Can you work these out from the model? Positions are in its coordinate system, mm. Round coordinates to 2 decimals unless told otherwise and drop trailing zeros. Loops run counter-clockwise (first coordinate to the right, second up) from the corner with the lowest first, then second, coordinate; pieces in that order, holes last. Notation, with made-up numbers: M 24,22.5 L 40,22.5 A36 cw 40,56.5 Z; hole C 19,9 d8. An arc over 180 degrees is marked long. Return JSON: item names as keys, results as strings.
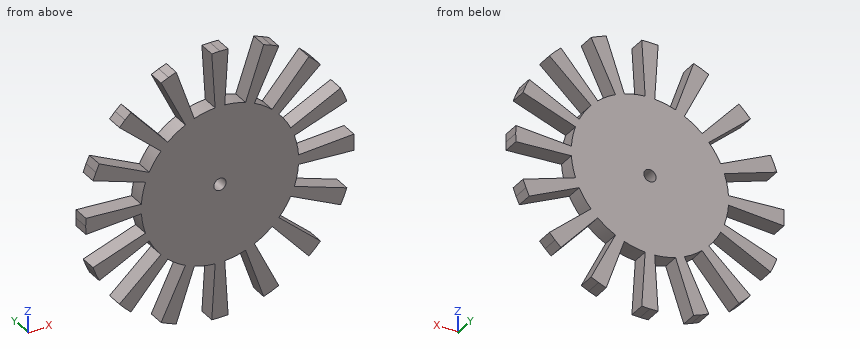
```python
from build123d import *

# Parameters (mm, degrees)
SKETCH2_R           = 1.89865
BOSS_EXTRUDE1_DEPTH = 5.1308


with BuildPart() as part:
    # Sketch2 → Boss-Extrude1 (new body)
    with BuildSketch(Plane(origin=(0, 0, 0), x_dir=(1, 0, 0), z_dir=(0, 1, 0))):
        with BuildLine():
            Line((-15.989661855, 38.602458507), (-13.614547531, 39.502698446))
            Line((-13.614547531, 39.502698446), (-7.982511303, 23.161308603))
            ThreePointArc((-7.982511303, 23.161308603), (-4.779381236, 24.027572035), (-1.488570263, 24.453033788))
            Line((-1.488570263, 24.453033788), (-2.538826421, 41.705796353))
            Line((-2.538826421, 41.705796353), (0, 41.783))
            Line((0, 41.783), (2.538826421, 41.705796353))
            Line((2.538826421, 41.705796353), (1.488570263, 24.453033788))
            ThreePointArc((1.488570263, 24.453033788), (4.779381236, 24.027572035), (7.982511303, 23.161308603))
            Line((7.982511303, 23.161308603), (13.614547531, 39.502698446))
            Line((13.614547531, 39.502698446), (15.989661855, 38.602458507))
            Line((15.989661855, 38.602458507), (18.305687065, 37.559564828))
            Line((18.305687065, 37.559564828), (10.733030501, 22.022006247))
            ThreePointArc((10.733030501, 22.022006247), (13.61052624, 20.369592003), (16.238327885, 18.34348414))
            Line((16.238327885, 18.34348414), (27.695230037, 31.285672794))
            Line((27.695230037, 31.285672794), (29.545042638, 29.545042638))
            Line((29.545042638, 29.545042638), (31.285672794, 27.695230037))
            Line((31.285672794, 27.695230037), (18.34348414, 16.238327885))
            ThreePointArc((18.34348414, 16.238327885), (20.369592003, 13.61052624), (22.022006247, 10.733030501))
            Line((22.022006247, 10.733030501), (37.559564828, 18.305687065))
            Line((37.559564828, 18.305687065), (38.602458507, 15.989661855))
            Line((38.602458507, 15.989661855), (39.502698446, 13.614547531))
            Line((39.502698446, 13.614547531), (23.161308603, 7.982511303))
            ThreePointArc((23.161308603, 7.982511303), (24.027572035, 4.779381236), (24.453033788, 1.488570263))
            Line((24.453033788, 1.488570263), (41.705796353, 2.538826421))
            Line((41.705796353, 2.538826421), (41.783, 0))
            Line((41.783, 0), (41.705796353, -2.538826421))
            Line((41.705796353, -2.538826421), (24.453033788, -1.488570263))
            ThreePointArc((24.453033788, -1.488570263), (24.027572035, -4.779381236), (23.161308603, -7.982511303))
            Line((23.161308603, -7.982511303), (39.502698446, -13.614547531))
            Line((39.502698446, -13.614547531), (38.602458507, -15.989661855))
            Line((38.602458507, -15.989661855), (37.559564828, -18.305687065))
            Line((37.559564828, -18.305687065), (22.022006247, -10.733030501))
            ThreePointArc((22.022006247, -10.733030501), (20.369592003, -13.61052624), (18.34348414, -16.238327885))
            Line((18.34348414, -16.238327885), (31.285672794, -27.695230037))
            Line((31.285672794, -27.695230037), (29.545042638, -29.545042638))
            Line((29.545042638, -29.545042638), (27.695230037, -31.285672794))
            Line((27.695230037, -31.285672794), (16.238327885, -18.34348414))
            ThreePointArc((16.238327885, -18.34348414), (13.61052624, -20.369592003), (10.733030501, -22.022006247))
            Line((10.733030501, -22.022006247), (18.305687065, -37.559564828))
            Line((18.305687065, -37.559564828), (15.989661855, -38.602458507))
            Line((15.989661855, -38.602458507), (13.614547531, -39.502698446))
            Line((13.614547531, -39.502698446), (7.982511303, -23.161308603))
            ThreePointArc((7.982511303, -23.161308603), (4.779381236, -24.027572035), (1.488570263, -24.453033788))
            Line((1.488570263, -24.453033788), (2.538826421, -41.705796353))
            Line((2.538826421, -41.705796353), (0, -41.783))
            Line((0, -41.783), (-2.538826421, -41.705796353))
            Line((-2.538826421, -41.705796353), (-1.488570263, -24.453033788))
            ThreePointArc((-1.488570263, -24.453033788), (-4.779381236, -24.027572035), (-7.982511303, -23.161308603))
            Line((-7.982511303, -23.161308603), (-13.614547531, -39.502698446))
            Line((-13.614547531, -39.502698446), (-15.989661855, -38.602458507))
            Line((-15.989661855, -38.602458507), (-18.305687065, -37.559564828))
            Line((-18.305687065, -37.559564828), (-10.733030501, -22.022006247))
            ThreePointArc((-10.733030501, -22.022006247), (-13.61052624, -20.369592003), (-16.238327885, -18.34348414))
            Line((-16.238327885, -18.34348414), (-27.695230037, -31.285672794))
            Line((-27.695230037, -31.285672794), (-29.545042638, -29.545042638))
            Line((-29.545042638, -29.545042638), (-31.285672794, -27.695230037))
            Line((-31.285672794, -27.695230037), (-18.34348414, -16.238327885))
            ThreePointArc((-18.34348414, -16.238327885), (-20.369592003, -13.61052624), (-22.022006247, -10.733030501))
            Line((-22.022006247, -10.733030501), (-37.559564828, -18.305687065))
            Line((-37.559564828, -18.305687065), (-38.602458507, -15.989661855))
            Line((-38.602458507, -15.989661855), (-39.502698446, -13.614547531))
            Line((-39.502698446, -13.614547531), (-23.161308603, -7.982511303))
            ThreePointArc((-23.161308603, -7.982511303), (-24.027572035, -4.779381236), (-24.453033788, -1.488570263))
            Line((-24.453033788, -1.488570263), (-41.705796353, -2.538826421))
            Line((-41.705796353, -2.538826421), (-41.783, 0))
            Line((-41.783, 0), (-41.705796353, 2.538826421))
            Line((-41.705796353, 2.538826421), (-24.453033788, 1.488570263))
            ThreePointArc((-24.453033788, 1.488570263), (-24.027572035, 4.779381236), (-23.161308603, 7.982511303))
            Line((-23.161308603, 7.982511303), (-39.502698446, 13.614547531))
            Line((-39.502698446, 13.614547531), (-38.602458507, 15.989661855))
            Line((-38.602458507, 15.989661855), (-37.559564828, 18.305687065))
            Line((-37.559564828, 18.305687065), (-22.022006247, 10.733030501))
            ThreePointArc((-22.022006247, 10.733030501), (-20.369592003, 13.61052624), (-18.34348414, 16.238327885))
            Line((-18.34348414, 16.238327885), (-31.285672794, 27.695230037))
            Line((-31.285672794, 27.695230037), (-29.545042638, 29.545042638))
            Line((-29.545042638, 29.545042638), (-27.695230037, 31.285672794))
            Line((-27.695230037, 31.285672794), (-16.238327885, 18.34348414))
            ThreePointArc((-16.238327885, 18.34348414), (-13.61052624, 20.369592003), (-10.733030501, 22.022006247))
            Line((-10.733030501, 22.022006247), (-18.305687065, 37.559564828))
            Line((-18.305687065, 37.559564828), (-15.989661855, 38.602458507))
        make_face()
        with Locations(Location((0, 0, 0), (0, 0, 270))):
            Circle(SKETCH2_R, mode=Mode.SUBTRACT)
    extrude(amount=BOSS_EXTRUDE1_DEPTH)


solid = part.part
```
Q1. If I drill on line 1 along X through (y, z) = (1.55, 0); line 2 along Z through (x, y) = (27, 4.75); line 3 along X through (y, z) = (2.6, -18), over which ranges is the centre line in solid material (lowest first)?
Results:
{"line 1": "x = -41.78 to -1.9, 1.9 to 41.78", "line 2": "z = -30.5 to -23.9, -13.16 to -9.31, -1.64 to 1.64, 9.31 to 13.16, 23.9 to 30.5", "line 3": "x = -37.7 to -36.93, -20.33 to 20.33, 36.93 to 37.7"}
Q2. Suppose I cut it at A-A, the plane x = -35.5. Please give me the cut outline in (y, z).
Results:
{"outline": "M 0,-17.3 L 5.13,-17.3 L 5.13,-12.24 L 0,-12.24 Z; M 0,-2.16 L 5.13,-2.16 L 5.13,2.16 L 0,2.16 Z; M 0,12.24 L 5.13,12.24 L 5.13,17.3 L 0,17.3 Z"}
Q3. I'm going to push flat-ended pins straight in: pin 1 Ø3 at (y, z) = (0.5, 25.5) entering from -X; pin 2 Ø1 at (x, y) = (-1.5, 0.5) entering from -Z. Where does each tip first touch, or does it pass through?
Results:
{"pin 1": "stops at x = -30.5", "pin 2": "stops at z = -41.75"}
